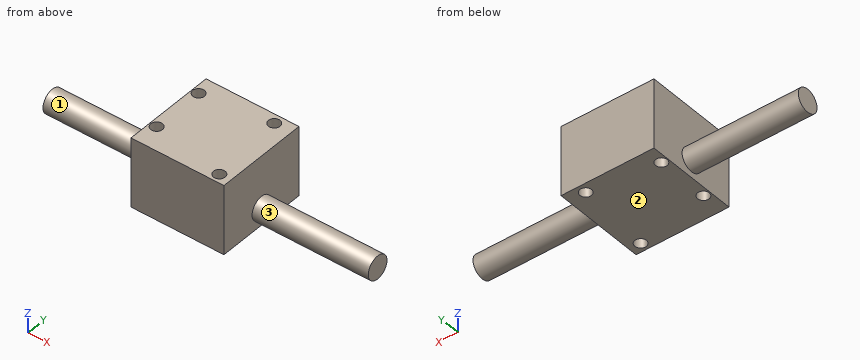
```python
from build123d import *

# Parameters (mm, degrees)
F0_W     = 50.8
F0_H     = 50.8
F0_R     = 3.175
F1_DEPTH = 19.05
F2_R     = 6.35
F3_DEPTH = 88.9


with BuildPart() as f1:
    # F0 (on Top) → F1 (new body, symmetric)
    with BuildSketch(Plane.XY):
        Rectangle(F0_W, F0_H)
        with Locations((-21.65604, -12.7)):
            Circle(F0_R, mode=Mode.SUBTRACT)
        with Locations((19.095719, -20.695919)):
            Circle(F0_R, mode=Mode.SUBTRACT)
        with Locations((-21.762719, 15.875)):
            Circle(F0_R, mode=Mode.SUBTRACT)
        with Locations((15.875, 20.482561)):
            Circle(F0_R, mode=Mode.SUBTRACT)
    extrude(amount=F1_DEPTH, both=True)

    # F2 (on Right) → F3 (join, symmetric)
    with BuildSketch(Plane.YZ):
        with Locations((0, -9.525)):
            Circle(F2_R)
    extrude(amount=F3_DEPTH, both=True)


solid = f1.part
```
The model under review builds one solid part; all positions refer to its coordinate system, in mm. Face numbers are marked on the shaded views. A direction names the side the tool comes from. Give positions to 0.01 mm unless a question says otherwise; leave off trailing zeros. Loops run counter-clockwise (first coordinate to the right, second up) from the corner with the lowest first, then second, coordinate; pieces in that order, holes last. Notation, with made-up numbers: (-16, 64) - (0, 64) arc R33 ccw to (0, 95) - close; hole circle Ø1 at (74.25, 39). An arc over 180 degrees is marked (long way). Answer as a JSON object with one key per item and string values.
Q1. Add section A-A on y = -12.7. State the section outline as (x, z) points.
Worked out:
{"outline": "(-25.4, -19.05) - (-24.83, -19.05) - (-24.83, 19.05) - (-25.4, 19.05) - close; (-18.48, -19.05) - (25.4, -19.05) - (25.4, 19.05) - (-18.48, 19.05) - close"}
Q2. Add section D-D on x = -52.5. State the section outline as (y, z) points (3 decimals), plus the area to 3 significant figures.
Worked out:
{"outline": "circle Ø12.7 at (0, -9.525)", "area": "127 mm^2"}
Q3. Insertion check: pin 1 (4 mm diameter, centred on x = 19.1, y = -20.7, fed in from +Z); pin 2 (5 mm diameter, centred on y = -13, z = -12, fed in from +X); pin 3 (5 mm diameter, centred on y = -7.5, z = 14, fed in from -X); pin 4 (12 mm diameter, centred on x = 34, z = -10.5, fed in from +Y). Each pin has a flat end and moves straight along its axis. Give the tip position at first contact, or say it passes through.
Worked out:
{"pin 1": "passes through", "pin 2": "stops at x = 25.4", "pin 3": "stops at x = -25.4", "pin 4": "stops at y = 6.35"}
Q4. Add section B-B on z = 11. State the section outline as (x, y) points (3 decimals).
Worked out:
{"outline": "(-25.4, -25.4) - (25.4, -25.4) - (25.4, 25.4) - (-25.4, 25.4) - close; hole circle Ø6.35 at (-21.763, 15.875); hole circle Ø6.35 at (-21.656, -12.7); hole circle Ø6.35 at (15.875, 20.483); hole circle Ø6.35 at (19.096, -20.696)"}
Q5. Add section C-C on y = 0. State the section outline as (x, z) points (3 decimals), plus the area to 3 significant figures.
Worked out:
{"outline": "(-88.9, -15.875) - (-25.4, -15.875) - (-25.4, -19.05) - (25.4, -19.05) - (25.4, -15.875) - (88.9, -15.875) - (88.9, -3.175) - (25.4, -3.175) - (25.4, 19.05) - (-25.4, 19.05) - (-25.4, -3.175) - (-88.9, -3.175) - close", "area": "3,550 mm^2"}
Q6. For the marked faces 1, 2 and 3, list the 3-axis set-ups (+Z, -Z, +X, -X, +Y, -Y) from which the entire face can be reached by the end or side of a thin tool; tool diameter is ignored.
Worked out:
{"face 1": "-X", "face 2": "-Z, +X, -X, +Y, -Y", "face 3": "+X"}
Q7. To check wall thickness, follow line 1 along Y through (x, z) = (-24, 3); line 2 along Y through (x, z) = (-20, 4.5); line 3 along Z through (x, y) = (75, 0) (3 decimals). State the ranges of each line that lie inside material, in increasing order.
Worked out:
{"line 1": "y = -25.4 to -14.84, -10.56 to 13.62, 18.13 to 25.4", "line 2": "y = -25.4 to -15.41, -9.99 to 13.23, 18.52 to 25.4", "line 3": "z = -15.875 to -3.175"}
